```python
from build123d import *
from OCP.BRepFilletAPI import BRepFilletAPI_MakeChamfer

# Parameters (mm, degrees)
SKETCH3_W           = 20
SKETCH3_H           = 40.6
BOSS_EXTRUDE1_DEPTH = 37
SKETCH3_3_W         = 20
SKETCH3_3_H         = 7.4
SKETCH3_3_R         = 2.25
BOSS_EXTRUDE2_DEPTH = 12.5
SKETCH3_4_W         = 20
SKETCH3_4_H         = 7.4
SKETCH3_4_R         = 2.25
CUT_EXTRUDE1_DEPTH  = 9.9
SKETCH3_5_R         = 3
SKETCH3_5_R_2       = 1
BOSS_EXTRUDE3_DEPTH = 6
SKETCH3_6_R         = 7.25
SKETCH3_6_R_2       = 3
BOSS_EXTRUDE4_DEPTH = 2
CHAMFER1_SIZE       = 4
CHAMFER1_SIZE2      = 2.309401077
CHAMFER3_SIZE       = 1.5
CHAMFER3_SIZE2      = 0.866025404
FILLET2_R           = 1
SKETCH4_W           = 6.858
SKETCH4_H           = 3.81
BOSS_EXTRUDE6_DEPTH = 2.5
CHAMFER4_SIZE       = 2.5
CHAMFER4_SIZE_2     = 0.5


with BuildPart() as part:
    # Sketch3 → Boss-Extrude1 (new body)
    with BuildSketch(Plane.XY):
        Rectangle(SKETCH3_W, SKETCH3_H)
    extrude(amount=-BOSS_EXTRUDE1_DEPTH)

    # Sketch3<3> → Boss-Extrude2 (add)
    # profile 1 of 2: a face of its own
    with BuildSketch(Plane.XY):
        with Locations((0, 24)):
            Rectangle(SKETCH3_3_W, SKETCH3_3_H)
        with Locations((-5, 24.3)):
            Circle(SKETCH3_3_R, mode=Mode.SUBTRACT)
        with Locations((5, 24.3)):
            Circle(SKETCH3_3_R, mode=Mode.SUBTRACT)
    # profile 2 of 2: a face of its own
    with BuildSketch(Plane.XY):
        Polygon((10, -20.3), (-10, -20.3), (-10, -27.7), (0, -27.7), (10, -27.7), align=None)
        with Locations((-5, -24.3)):
            Circle(SKETCH3_3_R, mode=Mode.SUBTRACT)
        with Locations((5, -24.3)):
            Circle(SKETCH3_3_R, mode=Mode.SUBTRACT)
    extrude(amount=-BOSS_EXTRUDE2_DEPTH)

    # Sketch3<4> → Cut-Extrude1 (cut)
    # profile 1 of 2: a face of its own
    with BuildSketch(Plane.XY):
        with Locations((0, 24)):
            Rectangle(SKETCH3_4_W, SKETCH3_4_H)
        with Locations((-5, 24.3)):
            Circle(SKETCH3_4_R, mode=Mode.SUBTRACT)
        with Locations((5, 24.3)):
            Circle(SKETCH3_4_R, mode=Mode.SUBTRACT)
    # profile 2 of 2: a face of its own
    with BuildSketch(Plane.XY):
        Polygon((10, -20.3), (-10, -20.3), (-10, -27.7), (0, -27.7), (10, -27.7), align=None)
        with Locations((-5, -24.3)):
            Circle(SKETCH3_4_R, mode=Mode.SUBTRACT)
        with Locations((5, -24.3)):
            Circle(SKETCH3_4_R, mode=Mode.SUBTRACT)
    extrude(amount=-CUT_EXTRUDE1_DEPTH, mode=Mode.SUBTRACT)

    # Sketch3<5> → Boss-Extrude3 (add)
    with BuildSketch(Plane.XY):
        with Locations((0, 9.8)):
            Circle(SKETCH3_5_R)
        with Locations((0, 9.8)):
            Circle(SKETCH3_5_R_2, mode=Mode.SUBTRACT)
    extrude(amount=BOSS_EXTRUDE3_DEPTH)

    # Sketch3<6> → Boss-Extrude4 (add)
    with BuildSketch(Plane.XY):
        with Locations((0, 9.8)):
            Circle(SKETCH3_6_R)
        with Locations((0, 9.8)):
            Circle(SKETCH3_6_R_2, mode=Mode.SUBTRACT)
    extrude(amount=BOSS_EXTRUDE4_DEPTH)

    # Chamfer1: one chamfer whose edges measure the first distance from different faces: ONE call of the kernel's chamfer builder (chamfer() names one face for all edges)
    chamfer1_edges_1 = [part.edges().sort_by_distance(p)[0] for p in [
        (10, 27.7, -11.2),
        (10, -27.7, -11.2),
    ]]
    chamfer1_side_1 = [part.faces().sort_by_distance(p)[0] for p in [
        (10, 0, -18.317675312),
    ]]
    chamfer1_edges_2 = [part.edges().sort_by_distance(p)[0] for p in [
        (-10, 27.7, -11.2),
        (-10, -27.7, -11.2),
    ]]
    chamfer1_side_2 = [part.faces().sort_by_distance(p)[0] for p in [
        (-10, 0, -18.317675312),
    ]]
    chamfer1 = BRepFilletAPI_MakeChamfer(part.part.solid().wrapped)
    for e in chamfer1_edges_1:
        chamfer1.Add(CHAMFER1_SIZE, CHAMFER1_SIZE2, e.wrapped, chamfer1_side_1[0].wrapped)  # the first distance lies on this face
    for e in chamfer1_edges_2:
        chamfer1.Add(CHAMFER1_SIZE, CHAMFER1_SIZE2, e.wrapped, chamfer1_side_2[0].wrapped)  # the first distance lies on this face
    add(Compound.cast(chamfer1.Shape()), mode=Mode.REPLACE)

    # Chamfer3
    chamfer3_edges = [part.edges().sort_by_distance(p)[0] for p in [
        (-7.25, 9.8, 2),
    ]]
    chamfer3_side = [part.faces().sort_by_distance(p)[0] for p in [
        (-7.25, 9.8, 1),
    ]]
    chamfer(chamfer3_edges, length=CHAMFER3_SIZE, length2=CHAMFER3_SIZE2, reference=chamfer3_side[0])

    # Fillet2
    fillet2_edges = [part.edges().sort_by_distance(p)[0] for p in [
        (10, -20.3, -24.75),
        (-10, -20.3, -24.75),
        (-10, 20.3, -24.75),
        (10, 20.3, -24.75),
        (-7.690598923, -27.7, -11.2),
        (7.690598923, -27.7, -11.2),
        (0, 20.3, -37),
        (10, 23.7, -11.2),
        (10, -23.7, -11.2),
        (-10, 23.7, -11.2),
        (-10, -23.7, -11.2),
        (-7.690598923, 27.7, -11.2),
        (7.690598923, 27.7, -11.2),
        (-6.383974596, 9.8, 2),
        (-10, 0, -37),
        (0, -20.3, -37),
        (10, 0, -37),
        (10, 0, 0),
        (-10, 0, 0),
        (10, 20.3, -4.95),
        (-10, 20.3, -4.95),
        (0, 20.3, 0),
        (10, -20.3, -4.95),
        (0, -20.3, 0),
        (-10, -20.3, -4.95),
    ]]
    fillet(fillet2_edges, radius=FILLET2_R)

    # Sketch4 → Boss-Extrude6 (add)
    with BuildSketch(Plane(origin=(0, 20.3, 0), x_dir=(1, 0, 0), z_dir=(0, 1, 0))):
        with Locations((0, 34.095)):
            Rectangle(SKETCH4_W, SKETCH4_H)
    extrude(amount=BOSS_EXTRUDE6_DEPTH)

    # Chamfer4
    chamfer4_edges_1 = [part.edges().sort_by_distance(p)[0] for p in [
        (0, 22.8, -32.19),
    ]]
    chamfer4_side_1 = [part.faces().sort_by_distance(p)[0] for p in [
        (0, 22.79, -32.19),
    ]]
    chamfer4_edges_2 = [part.edges().sort_by_distance(p)[0] for p in [
        (-3.429, 22.8, -34.095),
    ]]
    chamfer4_side_2 = [part.faces().sort_by_distance(p)[0] for p in [
        (-3.429, 22.79, -34.095),
    ]]
    chamfer4_edges_3 = [part.edges().sort_by_distance(p)[0] for p in [
        (0, 22.8, -36),
    ]]
    chamfer4_side_3 = [part.faces().sort_by_distance(p)[0] for p in [
        (0, 22.79, -36),
    ]]
    chamfer4_edges_4 = [part.edges().sort_by_distance(p)[0] for p in [
        (3.429, 22.8, -34.095),
    ]]
    chamfer4_side_4 = [part.faces().sort_by_distance(p)[0] for p in [
        (3.429, 22.79, -34.095),
    ]]
    chamfer4 = BRepFilletAPI_MakeChamfer(part.part.solid().wrapped)
    for e in chamfer4_edges_1:
        chamfer4.Add(CHAMFER4_SIZE - 0.0001, CHAMFER4_SIZE_2 - 0.0001, e.wrapped, chamfer4_side_1[0].wrapped)
    for e in chamfer4_edges_2:
        chamfer4.Add(CHAMFER4_SIZE - 0.0001, CHAMFER4_SIZE_2 - 0.0001, e.wrapped, chamfer4_side_2[0].wrapped)
    for e in chamfer4_edges_3:
        chamfer4.Add(CHAMFER4_SIZE - 0.0001, CHAMFER4_SIZE_2 - 0.0001, e.wrapped, chamfer4_side_3[0].wrapped)
    for e in chamfer4_edges_4:
        chamfer4.Add(CHAMFER4_SIZE - 0.0001, CHAMFER4_SIZE_2 - 0.0001, e.wrapped, chamfer4_side_4[0].wrapped)
    add(Compound.cast(chamfer4.Shape()), mode=Mode.REPLACE)  # a hair under: the kernel refuses the full size


solid = part.part
```
Part model, mm, in its own coordinate system. A direction names the side the tool comes from. Round coordinates to 2 decimals unless told otherwise and drop trailing zeros. Write each loop counter-clockwise with the first axis right and the second up, starting at its lowest first coordinate (ties: lowest second). Pieces come first, ordered by that corner, then holes. Notation, with made-up numbers: (50, 58.25) -> (65, 58.25) arc R17 ccw to (65, 80.25) -> close; hole circle Ø1 at (-24.75, 23). An arc over 180 degrees is marked (long way). Return JSON: item names as keys, results as strings. Group by question number.
Q1. Saw through at A-A on y = -6. Write the cut outline in (x, z), plus the area to 3 significant figures.
Q2. Saw through at B-B on z = -19. Write the cut outline in (x, y), plus the area to 3 significant figures.
Q3. Mould opens along X. For faces 4 (the flat face through (-8.91, -25.59, -11.18)), 5 (the flat face through (0, -23, -9.9)), 6 (the flat face through (0, 10, 0)) say: pulls with the +X half, pulls with the -X half, needs draft (parallel to the pull), parting line crosses it, or undercut.
Q4. Probe L1, parallel to Y at x = -5, z = -10.6; L2, parallel to X at y = 24, z = -11; L3, parallel to X at y = 23, z = -10.5. List the from-to ranges inside material, lowest first. Write a range as [from, to].
Q5. Saw through at D-D on x = -4.25. State how many separate pieces and enclosed holes the cut face has, plus the area to 3 significant figures.
Q6. Which spindle directions (+Z, -Z, +X, -X, +Y, -Y) get a long thin tool onto all of the face, cutting with end or side? Do faces 1 (the flat face through (3.176, 21.568, -34.068)), 2 (the flat face through (0, -20.3, -24)), 3 (the flat face through (0, 22.8, -34)). Say none if no direction does.
Q7. Pin check, flat tips, straight feed: pin 1 (8 mm diameter, centred on x = -3, y = 1, fed in from +Z); pin 2 (4 mm diameter, centred on x = 5, y = 24.3, fed in from +Z); pin 3 (1.4 mm diameter, centred on x = 0, z = -34, fed in from +Y); pin 4 (1 mm diameter, centred on x = -2.5, y = 17.5, fed in from +Z). Stop position of each tip, or through.
Q8. Saw through at C-C on y = 9.8. Write the cut outline in (x, z), plus the area to 3 significant figures.
Answer:
{
 "1": {"outline": "(-10, -36) arc R1 ccw to (-9, -37) -> (9, -37) arc R1 ccw to (10, -36) -> (10, -1) arc R1 ccw to (9, 0) -> (-9, 0) arc R1 ccw to (-10, -1) -> close", "area": "739 mm2"},
 "2": {"outline": "(-10, -19.3) arc R1 ccw to (-9, -20.3) -> (9, -20.3) arc R1 ccw to (10, -19.3) -> (10, 19.3) arc R1 ccw to (9, 20.3) -> (-9, 20.3) arc R1 ccw to (-10, 19.3) -> close", "area": "811 mm2"},
 "3": {"face 4": "pulls with the -X half", "face 5": "needs draft", "face 6": "undercut"},
 "4": {"L1": "[-27.7, -26.55], [-22.05, 22.05], [26.55, 27.7]", "L2": "[-9.83, -7.23], [-2.77, 2.77], [7.23, 9.83]", "L3": "[-10, -6.84], [-3.16, 3.16], [6.84, 10]"},
 "5": {"separate pieces": "3", "enclosed holes": "0", "area": "1,540 mm2"},
 "6": {"face 1": "-Z, +X, +Y", "face 2": "-Z, +X, -X, -Y", "face 3": "-Z, +X, -X, +Y"},
 "7": {"pin 1": "z = 2", "pin 2": "through", "pin 3": "y = 22.8", "pin 4": "z = 0"},
 "8": {"outline": "(-10, -36) arc R1 ccw to (-9, -37) -> (9, -37) arc R1 ccw to (10, -36) -> (10, -1) arc R1 ccw to (9, 0) -> (7.25, 0) -> (7.25, 0.5) -> (6.67, 1.5) arc R1 ccw to (5.81, 2) -> (3, 2) -> (3, 6) -> (1, 6) -> (1, 0) -> (-1, 0) -> (-1, 6) -> (-3, 6) -> (-3, 2) -> (-5.81, 2) arc R1 ccw to (-6.67, 1.5) -> (-7.25, 0.5) -> (-7.25, 0) -> (-9, 0) arc R1 ccw to (-10, -1) -> close", "area": "779 mm2"}
}
